```python
from build123d import *

# Parameters (mm, degrees)
F0_W        = 50
F0_H        = 50
F1_DEPTH    = 50
F2_R        = 21.0892085761
F4_DEPTH    = 50.001
F3_T1_DEPTH = 75


# Not quite as in the source:
# - a fillet or chamfer that OpenCascade refuses, or shapes differently, is made with other operations: its cross-section is extruded or revolved along the edge and cut away or added


with BuildPart() as f1:
    # F0 (on Top) → F1 (new body)
    with BuildSketch(Plane.XY):
        Rectangle(F0_W, F0_H)
    extrude(amount=F1_DEPTH)

    # F2 (on face) → F4 (cut, through all)
    with BuildSketch(Plane(origin=(-25, 0, 0), x_dir=(0, -1, 0), z_dir=(-1, 0, 0))):
        with Locations((0, 25.2627544105)):
            Circle(F2_R)
    extrude(amount=-F4_DEPTH, mode=Mode.SUBTRACT)

    # F3: fillet of radius 5 on 1 edges, made by hand

    # F3_s2 → F3_t1 (cut)
    with BuildSketch(Plane.XZ.offset(-37.5)):
        with BuildLine():
            ThreePointArc((25, 5), (23.5355339059, 1.4644660941), (20, 0))
            Line((20, 0), (25, 0))
            Line((25, 0), (25, 5))
        make_face()
    extrude(amount=F3_T1_DEPTH, mode=Mode.SUBTRACT)


solid = f1.part
```
The listing builds one solid part. Answer for the finished solid, in the listing's coordinates (mm). Coordinates: 2 decimals unless noted, no trailing zeros. Write each loop counter-clockwise with the first axis right and the second up, starting at its lowest first coordinate (ties: lowest second). Pieces come first, ordered by that corner, then holes. Notation, with made-up numbers: (10, 53.5) - (27, 53.5) arc R31 cw to (27, 86.5) - close; hole circle Ø7 at (52.5, 40.25). An arc over 180 degrees is marked (long way). Return JSON: item names as keys, results as strings. Group by question number.
Q1. The part is cut by section A-A on z = 6. Write down the section's boundary in (x, y).
Q2. Find the intervals of material crossed by line 1 along Y through (x, z) = (17.5, 25); line 2 along Z through (x, y) = (-7, 0); line 3 along Y through (x, z) = (9, 17), in increasing order. Write a range as [from, to].
Q3. The part is cut by section B-B on y = -7. Write down the section's boundary in (x, z), and give its area (3 significant figures).
Q4. A flat-ended cylindrical pin translates along its axis: pin 1 Ø10 at (y, z) = (6.5, 11) entering from -X. Find the tip coordinate at first contact, or state that the pin passes through.
Q5. The part is cut by section D-D on x = -1.5. Write down the section's boundary in (y, z).
Q6. The part is cut by section C-C on z = 23.5. Write down the section's boundary in (x, y).
Q7. For a pull along Z with two mould halves and no side action, classify faces 1 (the cylindrical face through (-0.35, 4.572, 4.675)), 2 (the flat face through (25, 0, 47)), 3 (the flat face through (0, 0, 50)) as +Z half, -Z half, draft (parallel to the pull), parting line (faces both ways), or undercut.
Evaluation:
{
 "1": {"outline": "(-25, -25) - (25, -25) - (25, -8.58) - (-25, -8.58) - close; (-25, 8.58) - (25, 8.58) - (25, 25) - (-25, 25) - close"},
 "2": {"line 1": "y = [-25, -21.09], [21.09, 25]", "line 2": "z = [0, 4.17], [46.35, 50]", "line 3": "y = [-25, -19.4], [19.4, 25]"},
 "3": {"outline": "(-25, 0) - (20, 0) arc R5 ccw to (25, 5) - (25, 5.37) - (-25, 5.37) - close; (-25, 45.16) - (25, 45.16) - (25, 50) - (-25, 50) - close", "area": "505 mm2"},
 "4": {"pin 1": "passes through"},
 "5": {"outline": "(-25, 0) - (25, 0) - (25, 50) - (-25, 50) - close; hole circle Ø42.18 at (0, 25.26)"},
 "6": {"outline": "(-25, -25) - (25, -25) - (25, -21.02) - (-25, -21.02) - close; (-25, 21.02) - (25, 21.02) - (25, 25) - (-25, 25) - close"},
 "7": {"face 1": "undercut", "face 2": "draft", "face 3": "+Z half"}
}
